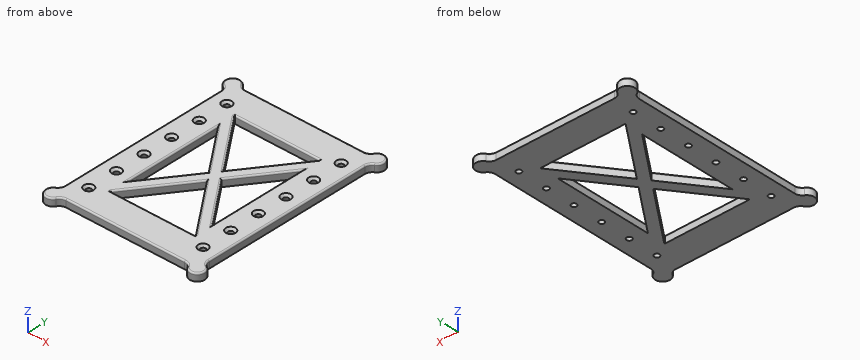
```python
from build123d import *

# Parameters (mm, degrees)
F0_R     = 1.75
F1_DEPTH = 5
F2_SIZE  = 1.5
F3_R     = 5
F5_R     = 1


with BuildPart() as f1:
    # F0 (on Top) → F1 (new body)
    with BuildSketch(Plane.XY):
        with BuildLine():
            ThreePointArc((0, 5), (-3.5355339059, -3.5355339059), (5, 0))
            Line((5, 0), (91.6, 0))
            ThreePointArc((91.6, 0), (100.1355339059, -3.5355339059), (96.6, 5))
            Line((96.6, 5), (96.6, 125))
            ThreePointArc((96.6, 125), (100.1355339059, 133.5355339059), (91.6, 130))
            Line((91.6, 130), (5, 130))
            ThreePointArc((5, 130), (-3.5355339059, 133.5355339059), (0, 125))
            Line((0, 125), (0, 5))
        make_face()
        with Locations((10, 15)):
            Circle(F0_R, mode=Mode.SUBTRACT)
        with Locations((10, 35)):
            Circle(F0_R, mode=Mode.SUBTRACT)
        with Locations((10, 55)):
            Circle(F0_R, mode=Mode.SUBTRACT)
        Polygon((20, 62.5), (20, 67.5), (20, 97.7074235808), (42.136, 67.5), (43.968, 65), (42.136, 62.5), (20, 32.2925764192), align=None, mode=Mode.SUBTRACT)
        with Locations((86.6, 15)):
            Circle(F0_R, mode=Mode.SUBTRACT)
        Polygon((76.6, 20), (20, 20), (20, 20.4694323144), (45.8, 55.6768558952), (48.3, 59.0884279476), (50.8, 55.6768558952), (76.6, 20.4694323144), align=None, mode=Mode.SUBTRACT)
        Polygon((76.6, 97.7074235808), (76.6, 67.5), (76.6, 62.5), (76.6, 32.2925764192), (54.464, 62.5), (52.632, 65), (54.464, 67.5), align=None, mode=Mode.SUBTRACT)
        with Locations((86.6, 35)):
            Circle(F0_R, mode=Mode.SUBTRACT)
        with Locations((86.6, 55)):
            Circle(F0_R, mode=Mode.SUBTRACT)
        with Locations((10, 75)):
            Circle(F0_R, mode=Mode.SUBTRACT)
        with Locations((10, 95)):
            Circle(F0_R, mode=Mode.SUBTRACT)
        with Locations((10, 115)):
            Circle(F0_R, mode=Mode.SUBTRACT)
        Polygon((20, 109.5305676856), (20, 110), (45.8, 110), (50.8, 110), (76.6, 110), (76.6, 109.5305676856), (50.8, 74.3231441048), (48.3, 70.9115720524), (45.8, 74.3231441048), align=None, mode=Mode.SUBTRACT)
        with Locations((86.6, 75)):
            Circle(F0_R, mode=Mode.SUBTRACT)
        with Locations((86.6, 95)):
            Circle(F0_R, mode=Mode.SUBTRACT)
        with Locations((86.6, 115)):
            Circle(F0_R, mode=Mode.SUBTRACT)
    extrude(amount=F1_DEPTH)

    # F2
    f2_edges = [f1.edges().sort_by_distance(p)[0] for p in [
        (8.25, 15, 5),
        (8.25, 35, 5),
        (8.25, 55, 5),
        (8.25, 75, 5),
        (8.25, 95, 5),
        (8.25, 115, 5),
        (84.85, 115, 5),
        (84.85, 95, 5),
        (84.85, 75, 5),
        (84.85, 55, 5),
        (84.85, 35, 5),
        (84.85, 15, 5),
    ]]
    chamfer(f2_edges, length=F2_SIZE)

    # F3
    f3_edges = [f1.edges().sort_by_distance(p)[0] for p in [
        (5, 0, 2.5),
        (91.6, 0, 2.5),
        (96.6, 5, 2.5),
        (96.6, 125, 2.5),
        (91.6, 130, 2.5),
        (5, 130, 2.5),
        (0, 125, 2.5),
        (0, 5, 2.5),
    ]]
    fillet(f3_edges, radius=F3_R)

    # F5
    f5_edges = [f1.edges().sort_by_distance(p)[0] for p in [
        (48.3, 0, 5),
        (100.135534, -3.535534, 5),
        (90.439746, -0.669873, 5),
        (97.269873, 6.160254, 5),
        (96.6, 65, 5),
        (97.269873, 123.839746, 5),
        (100.135534, 133.535534, 5),
        (90.439746, 130.669873, 5),
        (48.3, 130, 5),
        (6.160254, 130.669873, 5),
        (-3.535534, 133.535534, 5),
        (-0.669873, 123.839746, 5),
        (0, 65, 5),
        (-0.669873, 6.160254, 5),
        (-3.535534, -3.535534, 5),
        (6.160254, -0.669873, 5),
        (31.984, 81.353712, 5),
        (20, 65, 5),
        (31.984, 48.646288, 5),
        (34.15, 90.22107, 5),
        (62.45, 90.22107, 5),
        (48.3, 110, 5),
        (64.616, 48.646288, 5),
        (64.616, 81.353712, 5),
        (76.6, 65, 5),
        (62.45, 39.77893, 5),
        (34.15, 39.77893, 5),
        (48.3, 20, 5),
        (20, 20.234716, 5),
        (76.6, 20.234716, 5),
        (76.6, 109.765284, 5),
        (20, 109.765284, 5),
    ]]
    fillet(f5_edges, radius=F5_R)


solid = f1.part
```
Can you work these out from the model? Positions are in its coordinate system, mm. Coordinates: 2 decimals unless noted, no trailing zeros. Loops run counter-clockwise (first coordinate to the right, second up) from the corner with the lowest first, then second, coordinate; pieces in that order, holes last. Notation, with made-up numbers: (59.25, 20) -> (112.25, 20) arc R24 ccw to (112.25, 59) -> close; hole circle Ø1 at (77, 34). An arc over 180 degrees is marked (long way). Put each result on its own line as item: value. Start each with the question number.
Q1. I want a section at A-A (y = 15). Write out the boundary of the cut face in (x, z), plus the area to 3 significant figures.
Q2. I want a section at B-B (z = 2.4). Count the separate pieces of the cut face and the enclosed holes in it, plus the area to 3 significant figures.
Q3. If I drill on line 1 (X direction, y = 115, z = 1.25); line 2 (Y direction, x = 59.5, z = 1); line 3 (X direction, y = 39, z = 0.4), over which ranges is the centre line in solid material (lowest first)? Write a range as [from, to].
Q4. I'm going to push flat-ended pins straight in: P1, Ø5.5, axis at x = 10, y = 35, coming from the +Z side; P2, Ø1, axis at x = 70.5, z = 3.5, coming from the -Y side; P3, Ø3, axis at y = 84.5, z = 2.5, coming from the -X side; P4, Ø3, axis at x = 86.6, y = 55, coming from the +Z side. Where does each tip first touch, or does it pass through?
Taken from the geometry:
1. outline: (0, 0) -> (8.25, 0) -> (8.25, 3.5) -> (6.75, 5) -> (1, 5) arc R1 ccw to (0, 4) -> close; (11.75, 0) -> (84.85, 0) -> (84.85, 3.5) -> (83.35, 5) -> (13.25, 5) -> (11.75, 3.5) -> close; (88.35, 0) -> (96.6, 0) -> (96.6, 4) arc R1 ccw to (95.6, 5) -> (89.85, 5) -> (88.35, 3.5) -> close
1. area: 443 mm2
2. separate pieces: 1
2. enclosed holes: 16
2. area: 8,890 mm2
3. line 1: x = [0, 8.25], [11.75, 84.85], [88.35, 96.6]
3. line 2: y = [0, 20], [43.8, 55.63], [74.37, 86.2], [110, 130]
3. line 3: x = [0, 20], [24.92, 33.58], [63.02, 71.68], [76.6, 96.6]
4. P1: stops at z = 4.5
4. P2: stops at y = 0
4. P3: stops at x = 0
4. P4: passes through
